```python
from build123d import *

# Parameters (mm, degrees)
BOSS_EXTRUDE2_DEPTH = 5
SKETCH7_R           = 4.75
CUT_EXTRUDE1_DEPTH  = 19.75
SKETCH8_R           = 5
CUT_EXTRUDE2_DEPTH  = 132.5


with BuildPart() as part:
    # Sketch1 → Revolve2 (revolve)
    with BuildSketch(Plane.XY):
        Polygon((157.5, 0), (0, 0), (0, 13.75), (31.25, 13.15), (31.25, 11.25), (157.5, 8.75), align=None)
    revolve(axis=Axis((157.5, 0, 0), (-1, 0, 0)))

    # Sketch2 → Boss-Extrude2 (add, symmetric)
    with BuildSketch(Plane.XY):
        with BuildLine():
            Line((157.5, 8.75), (174.296707174, 8.417391937))
            ThreePointArc((174.296707174, 8.417391937), (182.618377126, 0), (174.296707174, -8.417391937))
            Line((174.296707174, -8.417391937), (157.5, -8.75))
            Line((157.5, -8.75), (157.5, 8.75))
        make_face()
    extrude(amount=BOSS_EXTRUDE2_DEPTH, both=True)

    # Sketch6 → Cut-Revolve1 (revolve, cut)
    with BuildSketch(Plane.XY):
        Polygon((157.5, 8.75), (157.5, 12.5), (189.266018866, 12.5), (189.266018866, 8.120969923), align=None)
    revolve(axis=Axis((157.5, 0, 0), (1, 0, 0)), mode=Mode.SUBTRACT)

    # Sketch7 → Cut-Extrude1 (cut, through all)
    with BuildSketch(Plane.XY.offset(5)):
        with Locations((170.368377126, 0)):
            Circle(SKETCH7_R)
    extrude(amount=-CUT_EXTRUDE1_DEPTH, mode=Mode.SUBTRACT)

    # Sketch8 → Cut-Extrude2 (cut)
    with BuildSketch(Plane.ZY):
        Circle(SKETCH8_R)
    extrude(amount=-CUT_EXTRUDE2_DEPTH, mode=Mode.SUBTRACT)


solid = part.part
```
Read the model definition and answer for the solid it produces. Units are mm, in the model's axes. A direction names the side the tool comes from. Give positions to 0.01 mm unless a question says otherwise; leave off trailing zeros. Order: outer loops, then holes, each group sorted by start corner. A loop starts at its lowest first (then second) coordinate and runs counter-clockwise, first axis right, second up. Notation, with made-up numbers: (40.25, -13) -> (77.25, -13) arc R32 ccw to (77.25, 17) -> close; hole circle Ø10 at (-20, -20.75). An arc over 180 degrees is marked (long way). Write item = value, one per line.
1. A cutting plane is placed at A-A, the plane x = 42. Write down the section's boundary in (y, z).
Numbers:
outline = circle Ø22.07 at (0, 0); hole circle Ø10 at (0, 0)
2. A cutting plane is placed at C-C, the plane x = 69.5. Write down the section's boundary in (y, z).
Numbers:
outline = circle Ø20.99 at (0, 0); hole circle Ø10 at (0, 0)
3. A cutting plane is placed at B-B, the plane x = 145. Write down the section's boundary in (y, z), and give its area (3 significant figures).
Numbers:
outline = circle Ø18 at (0, 0)
area = 254 mm²
4. Given pin 1 (1 mm diameter, centred on y = -1, z = 0, fed in from -X); pin 2 (8.5 mm diameter, centred on x = 170.37, y = 0, fed in from -Z); pin 3 (3 mm diameter, centred on x = 79.5, y = 3, fed in from +Z); pin 4 (6 mm diameter, centred on x = 142, y = -10, fed in from -Z), each flat-ended and moving along its own axis, determine where each tip first touches the part or whether it passes through.
Numbers:
pin_1 = 132.5
pin_2 = through
pin_3 = 10.19
pin_4 = -5.75
5. The mould has two halves that part along X. Classify faces 1 (the face through (31.25, 10, -6)), 2 (the face through (170, 5, 5)), 3 (the face through (165.623, 0.209, 0.07)): +X half, -X half, draft (parallel to the pull), parting line (faces both ways), or undercut.
Numbers:
face_1 = +X half
face_2 = draft
face_3 = undercut
6. Straight lines are drawn through the part: line 1 along X through (y, z) = (11, 3.75); line 2 along X through (y, z) = (-4.75, 5.75); line 3 along Y through (x, z) = (97.5, -2.5). For each, find the intervals that lie inside material, in ascending order.
Numbers:
line_1 = 0 to 31.25
line_2 = 0 to 157.5
line_3 = -9.62 to -4.33, 4.33 to 9.62
7. For faces 4 (the face through (15.84, 6.2, 11.93)), 5 (the face through (157.5, 0, 6)), 6 (the face through (65.32, -4.88, -1.08)), 7 (the face through (157.5, 0, -6)), determine the directions among +Z, -Z, +X, -X, +Y, -Y from which every point of the face is accessible in a straight line to the end or side of a thin tool.
Numbers:
face_4 = +X
face_5 = +Z, +X, +Y, -Y
face_6 = -X
face_7 = -Z, +X, +Y, -Y
